```python
from build123d import *

# Parameters (mm, degrees)
BOSS_EXTRUDE1_DEPTH = 3.96875
SKETCH4_OUTSIDE_W   = 616.832
SKETCH4_OUTSIDE_H   = 618.552
SKETCH4_OUTSIDE_R   = 5.000625
CUT_EXTRUDE1_DEPTH  = 233.723565508
CUT_EXTRUDE1_DRAFT  = -50
SKETCH9_R           = 6.415804866
SKETCH9_R_2         = 5.2784375
CUT_EXTRUDE2_DEPTH  = 0.09921875


with BuildPart() as part:
    # Sketch2 → Revolve1 (revolve)
    with BuildSketch(Plane(origin=(0, 0, 0), x_dir=(0, 0, -1), z_dir=(1, 0, 0)), mode=Mode.PRIVATE) as revolve1_sk:
        Polygon((228.6, 0), (0, 0), (0, 3.175), (227.711, 3.175), (228.6, 2.286), align=None)
    revolve(revolve1_sk.sketch.rotate(Axis((0, 0, -228.6), (0, 0, 1)), 90), axis=Axis((0, 0, -228.6), (0, 0, 1)))

    # Sketch3 → Boss-Extrude1 (add)
    with BuildSketch(Plane.XY):
        Polygon((0, 6.415804866), (-5.55625, 3.207902433), (-5.55625, -3.207902433), (0, -6.415804866), (5.55625, -3.207902433), (5.55625, 3.207902433), align=None)
    extrude(amount=BOSS_EXTRUDE1_DEPTH)


with BuildPart() as cut_extrude1_tool:
    # Sketch4 outside → Cut-Extrude1 (with draft: the straight prism first)
    with BuildSketch(Plane.XY.offset(3.96875)):
        Rectangle(SKETCH4_OUTSIDE_W, SKETCH4_OUTSIDE_H)
        Circle(SKETCH4_OUTSIDE_R, mode=Mode.SUBTRACT)
    extrude(amount=-CUT_EXTRUDE1_DEPTH)
    # Cut-Extrude1: the draft: its side faces are tilted about the plane it starts from
    cut_extrude1_sides = [cut_extrude1_tool.faces().sort_by_distance(p)[0] for p in [
        (0, -309.276, -112.893032754),
        (308.416, 0, -112.893032754),
        (0, 309.276, -112.893032754),
        (-308.416, 0, -112.893032754),
        (-5.000625, 0, -112.893032754),
    ]]
    draft(cut_extrude1_sides, Plane.XY.offset(3.96875), CUT_EXTRUDE1_DRAFT)


with BuildPart() as part_1:
    add(part.part)

    # Cut-Extrude1: cut by cut_extrude1_tool
    add(cut_extrude1_tool.part, mode=Mode.SUBTRACT)

    # Sketch9 → Cut-Extrude2 (cut)
    with BuildSketch(Plane(origin=(0, 0, 0), x_dir=(-1, 0, 0), z_dir=(0, 0, -1))):
        Circle(SKETCH9_R)
        Circle(SKETCH9_R_2, mode=Mode.SUBTRACT)
    extrude(amount=-CUT_EXTRUDE2_DEPTH, mode=Mode.SUBTRACT)


solid = part_1.part
```
Input: part model. Units: mm. Frame: model coordinates. A direction names the side the tool comes from. Coordinates: 2 decimals unless noted, no trailing zeros. Loops run counter-clockwise (first coordinate to the right, second up) from the corner with the lowest first, then second, coordinate; pieces in that order, holes last. Notation, with made-up numbers: M -36.75,-29.5 L 15.25,-29.5 A25 ccw 15.25,4.5 Z; hole C 72.25,17.25 d5. An arc over 180 degrees is marked long. Use a Markdown table: item, result. Add a question column.
1) Set-up query: faces 1 (the flat face through (0, 0, -228.6)), 2 (the cylindrical face through (2.52, 1.93, -115.45)). Return all of +Z, -Z, +X, -X, +Y, -Y with unobstructed straight access to the full face (end or side cutting, diameter ignored); none if empty.
2) Line query: L1, parallel to Z at x = 2.5, y = -2.75; L2, parallel to X at y = 2.25, z = -85; L3, parallel to X at y = -0.5, z = -94. Output: solid intervals per line, ascending. Write a range as from..to.
3) Pin query (flat end, axial travel): P1, Ø4, axis at x = 4, z = -77.5, coming from the -Y side; P2, Ø6, axis at y = -3.5, z = -162, coming from the +X side; P3, Ø1.5, axis at x = -3.5, z = -100, coming from the +Y side. Return the tip coordinate at first contact, or that it passes through.
4) Section B-B, the plane z = -59.5. Return the cut outline in (x, y) (3 decimals).
5) Section A-A, the plane y = 0. Return the cut outline in (x, z) (3 decimals), plus the area to 3 significant figures.
Answer below:
| question | item | result |
|---|---|---|
| 1 | face 1 | -Z, +X, -X, +Y, -Y |
| 1 | face 2 | -Z |
| 2 | L1 | 0..3.97 |
| 2 | L2 | -2.24..2.24 |
| 2 | L3 | -3.14..3.14 |
| 3 | P1 | y = -2.47 |
| 3 | P2 | x = 3.14 |
| 3 | P3 | y = 1.59 |
| 4 | outline | C 0,0 d6.35 |
| 5 | outline | M -5.556,0.099 L -5.278,0.099 L -5.278,0 L -3.175,0 L -3.175,-227.711 L -2.286,-228.6 L 2.286,-228.6 L 3.175,-227.711 L 3.175,0 L 5.278,0 L 5.278,0.099 L 5.556,0.099 L 5.556,3.503 L 5.001,3.969 L -5.001,3.969 L -5.556,3.503 Z |
| 5 | area | 1,490 mm2 |
